Geometry: final body of the model. Coordinates: model frame, mm. A direction names the side the tool comes from. Round coordinates to 2 decimals unless told otherwise and drop trailing zeros. Loops run counter-clockwise (first coordinate to the right, second up) from the corner with the lowest first, then second, coordinate; pieces in that order, holes last. Notation, with made-up numbers: M 22.25,85 L 50.25,85 A21 ccw 50.25,89 Z; hole C -14.75,-34.75 d10. An arc over 180 degrees is marked long. Return JSON: item names as keys, results as strings.
from build123d import *

# Parameters (mm, degrees)
SKETCH_1_W          = 44
SKETCH_1_H          = 35
EXTRUDE_1_DEPTH     = 2
SKETCH_2_W          = 17
SKETCH_2_H          = 17
EXTRUDE_2_DEPTH     = 14
SKETCH_3_R          = 8
EXTRUDE_3_DEPTH     = 14
SKETCH_4_R          = 1.5
CUT_EXTRUDE_1_DEPTH = 10


with BuildPart() as part:
    # 草图1 → 凸台-拉伸1 (new body)
    with BuildSketch(Plane(origin=(0, 0, 0), x_dir=(1, 0, 0), z_dir=(0, 1, 0))):
        Rectangle(SKETCH_1_W, SKETCH_1_H)
    extrude(amount=EXTRUDE_1_DEPTH)

    # 草图2 → 凸台-拉伸2 (add)
    with BuildSketch(Plane(origin=(0, 2, 0), x_dir=(1, 0, 0), z_dir=(0, 1, 0))):
        with Locations((13.5, 0)):
            Rectangle(SKETCH_2_W, SKETCH_2_H)
    extrude(amount=EXTRUDE_2_DEPTH)

    # 草图3 → 凸台-拉伸3 (add)
    with BuildSketch(Plane(origin=(0, 16, 0), x_dir=(1, 0, 0), z_dir=(0, 1, 0))):
        with Locations(Location((13.5, 0, 0), (0, 0, 270))):
            Circle(SKETCH_3_R)
    extrude(amount=EXTRUDE_3_DEPTH)

    # 草图4 → 切除-拉伸1 (cut)
    with BuildSketch(Plane.XZ):
        with Locations(Location((16.511574999, -15, 0), (0, 0, 270))):
            Circle(SKETCH_4_R)
        with Locations(Location((16.511574999, 15, 0), (0, 0, 90))):
            Circle(SKETCH_4_R)
    extrude(amount=-CUT_EXTRUDE_1_DEPTH, mode=Mode.SUBTRACT)


solid = part.part
Q1. Material intervals for L1, parallel to X at y = 1.3, z = -15; L2, parallel to Y at x = -4, z = 7; L3, parallel to X at y = 9.25, z = 0, sorted ascending.
Determined:
{"L1": "x = -22 to 15.01, 18.01 to 22", "L2": "y = 0 to 2", "L3": "x = 5 to 22"}
Q2. Section query B-B (x = 13.5). Output: boundary loops of the cut face in (y, z).
Determined:
{"outline": "M 0,-17.5 L 2,-17.5 L 2,-8.5 L 16,-8.5 L 16,-8 L 30,-8 L 30,8 L 16,8 L 16,8.5 L 2,8.5 L 2,17.5 L 0,17.5 Z"}
Q3. Section query D-D (y = 19.75). Output: boundary loops of the cut face in (x, z).
Determined:
{"outline": "C 13.5,0 d16"}
Q4. Section query C-C (z = 0). Output: boundary loops of the cut face in (x, y), plus the area to 3 significant figures.
Determined:
{"outline": "M -22,0 L 22,0 L 22,16 L 21.5,16 L 21.5,30 L 5.5,30 L 5.5,16 L 5,16 L 5,2 L -22,2 Z", "area": "550 mm^2"}
Q5. Pin query (flat end, axial travel): pin 1 (1.5 mm diameter, centred on y = 23.5, z = 6.5, fed in from -X); pin 2 (4 mm diameter, centred on y = 19, z = -4, fed in from -X); pin 3 (3 mm diameter, centred on x = 3, z = -13, fed in from +Y). Return the tip coordinate at first contact, or that it passes through.
Determined:
{"pin 1": "stops at x = 7.94", "pin 2": "stops at x = 5.75", "pin 3": "stops at y = 2"}
Q6. Pull-direction query (Z, two-part tool) for faces 1 (the flat face through (13, 9, -8.5)), 2 (the flat face through (13, 9, 8.5)), 3 (the flat face through (11, 16, -8)), 4 (the cylindrical face through (16.45, 0.99, 13.5)); classes: pulls with the +Z half, pulls with the -Z half, needs draft (parallel to the pull), parting line crosses it, or undercut.
Determined:
{"face 1": "pulls with the -Z half", "face 2": "pulls with the +Z half", "face 3": "needs draft", "face 4": "undercut"}
Q7. Reachability of faces 5 (the flat face through (5, 9, 0)), 6 (the flat face through (14, 30, 0)), 7 (the cylindrical face through (13.852, 22.902, -7.992)) from +Z, -Z, +X, -X, +Y, -Y: full face, straight path, thin tool, end or side. Return the list, or none.
Determined:
{"face 5": "+Z, -Z, -X, +Y", "face 6": "+Z, -Z, +X, -X, +Y", "face 7": "+Y"}
Q8. Section query A-A (z = 15). Output: boundary loops of the cut face in (x, y).
Determined:
{"outline": "M -22,0 L 15.01,0 L 15.01,2 L -22,2 Z; M 18.01,0 L 22,0 L 22,2 L 18.01,2 Z"}
